from build123d import *

# Parameters (mm, degrees)
EXTRUDE1_DEPTH               = 10
EXTRUDE2_DEPTH               = 15
FILLET1_R                    = 8
SKETCH3_R                    = 2.5
CUT_EXTRUDE1_DEPTH           = 53.683044042
FILLET4_R                    = 8
FILLET7_R                    = 4
SKETCH4_W                    = 5
SKETCH4_H                    = 25.2
EXTRUDE3_DEPTH               = 117.395755978
F_4_0_4_DIAMETER_HOLE1_D     = 4
F_4_0_4_DIAMETER_HOLE1_DEPTH = 15
SKETCH6_W                    = 50
SKETCH6_H                    = 10
EXTRUDE4_DEPTH               = 22
SKETCH7_W                    = 35.991558426
SKETCH7_H                    = 19.258240123
EXTRUDE5_DEPTH               = 65
SKETCH8_R                    = 7
EXTRUDE6_DEPTH               = 65
SKETCH9_R                    = 11.25
EXTRUDE7_DEPTH               = 8
FILLET8_R                    = 10
SKETCH11_W                   = 10
SKETCH11_H                   = 24.2
EXTRUDE9_DEPTH               = 28
F_4_0_4_DIAMETER_HOLE2_D     = 4
F_4_0_4_DIAMETER_HOLE2_DEPTH = 15
SKETCH13_W                   = 8
SKETCH13_H                   = 22
CUT_EXTRUDE2_DEPTH           = 16
F_4_0_4_DIAMETER_HOLE3_D     = 3.9
F_4_0_4_DIAMETER_HOLE3_DEPTH = 15
EXTRUDE10_DEPTH              = 10
FILLET9_R                    = 5
FILLET10_R                   = 3


with BuildPart() as part:
    # Sketch1 → Extrude1 (new body)
    with BuildSketch(Plane.XY):
        Polygon((-68.067337579, -53.151608792), (46.932662421, -53.151608792), (46.932662421, -28.951608792), (56.08269406, -28.951608792), (56.08269406, -20.951608792), (46.932662421, -20.951608792), (46.932662421, 91.048391208), (36.605660332, 91.048391208), (25.932662421, 91.048391208), (25.932662421, 86.048391208), (36.932662421, 86.048391208), (36.932662421, 80.948391208), (25.932662421, 80.948391208), (25.932662421, 50.948391208), (36.932662421, 50.948391208), (36.932662421, 45.848391208), (25.932662421, 45.848391208), (25.932662421, 40.848391208), (36.932662421, 40.848391208), (36.932662421, 25.69350339), (36.932662421, 22.150468938), (36.932662421, 14.848391208), (-58.067337579, 14.848391208), (-58.067337579, -20.951608792), (-68.067337579, -20.951608792), align=None)
    extrude(amount=EXTRUDE1_DEPTH)

    # Sketch2 → Extrude2 (add)
    with BuildSketch(Plane.XY.offset(10)):
        Polygon((25.932662421, 91.048391208), (46.932662421, 91.048391208), (46.932662421, 41.227475545), (36.932662421, 41.227475545), (36.932662421, 40.848391208), (25.932662421, 40.848391208), (25.932662421, 45.848391208), (36.932662421, 45.848391208), (36.932662421, 50.948391208), (25.932662421, 50.948391208), (25.932662421, 80.948391208), (36.932662421, 80.948391208), (36.932662421, 86.048391208), (25.932662421, 86.048391208), align=None)
    extrude(amount=EXTRUDE2_DEPTH)

    # Fillet1
    fillet1_edges = [part.edges().sort_by_distance(p)[0] for p in [
        (25.932662421, 65.948391208, 0),
        (25.932662421, 65.948391208, 25),
    ]]
    fillet(fillet1_edges, radius=FILLET1_R)

    # Sketch3 → Cut-Extrude1 (cut)
    with BuildSketch(Plane(origin=(0, 91.048391208, 0), x_dir=(-1, 0, 0), z_dir=(0, 1, 0))):
        with Locations(Location((-30.932662421, 5.5, 0), (0, 0, 90))):
            Circle(SKETCH3_R)
        with Locations(Location((-30.932662421, 19.5, 0), (0, 0, 90))):
            Circle(SKETCH3_R)
    extrude(amount=-CUT_EXTRUDE1_DEPTH, mode=Mode.SUBTRACT)

    # Fillet4
    fillet4_edges = [part.edges().sort_by_distance(p)[0] for p in [
        (46.932662421, 91.048391208, 12.5),
    ]]
    fillet(fillet4_edges, radius=FILLET4_R)

    # Fillet7
    # the kernel refuses this fillet: 4 mm, written as the material it takes off along each edge
    with BuildSketch(Plane(origin=(46.932662421, 83.048391208, 25), x_dir=(-1, 0, 0), z_dir=(0, -1, 0))) as fillet7_piece_1:
        with BuildLine():
            CenterArc((FILLET7_R, FILLET7_R), FILLET7_R, 180, 90)
            Line((0, FILLET7_R), (0, 0))
            Line((0, 0), (FILLET7_R, 0))
        make_face()
    extrude(amount=51.820915662, mode=Mode.SUBTRACT)
    with BuildSketch(Plane(origin=(15.932662421, 91.048391208, 25), x_dir=(0, -1, 0), z_dir=(1, 0, 0))) as fillet7_piece_2:
        with BuildLine():
            CenterArc((FILLET7_R, FILLET7_R), FILLET7_R, 180, 90)
            Line((0, FILLET7_R), (0, 0))
            Line((0, 0), (FILLET7_R, 0))
        make_face()
    extrude(amount=23, mode=Mode.SUBTRACT)
    with BuildSketch(Plane(origin=(38.932662421, 83.048391208, 25), x_dir=(0, 1, 0), z_dir=(-1, 0, 0))) as fillet7_piece_3:
        with BuildLine():
            CenterArc((8 - FILLET7_R, FILLET7_R), FILLET7_R, 270, 90)
            Line((8, FILLET7_R), (8, 0))
            Line((8, 0), (8 - FILLET7_R, 0))
        make_face()
    revolve(axis=Axis((38.932662421, 83.048391208, 25), (0, 0, -1)), revolution_arc=90, mode=Mode.SUBTRACT)

    # Sketch4 → Extrude3 (cut, through all)
    with BuildSketch(Plane(origin=(0, 0, 0), x_dir=(-1, 0, 0), z_dir=(0, 0, -1))):
        with Locations((-44.432662421, 68.348391208)):
            Rectangle(SKETCH4_W, SKETCH4_H)
    extrude(amount=-EXTRUDE3_DEPTH, mode=Mode.SUBTRACT)

    # Ø4.0 (4) Diameter Hole1
    with Locations(Plane(origin=(41.932662421, 75.948391208, 12), x_dir=(0, 1, 0), z_dir=(1, 0, 0))):
        with Locations((0, 0), (-16, 0)):
            Hole(F_4_0_4_DIAMETER_HOLE1_D / 2, depth=F_4_0_4_DIAMETER_HOLE1_DEPTH)

    # Sketch6 → Extrude4 (add)
    with BuildSketch(Plane.XY.offset(10)):
        with Locations((-18.067337579, 9.848391208)):
            Rectangle(SKETCH6_W, SKETCH6_H)
    extrude(amount=EXTRUDE4_DEPTH)

    # Sketch7 → Extrude5 (cut)
    with BuildSketch(Plane.XY.offset(10)):
        with Locations((-17.995779213, -4.780728854)):
            Rectangle(SKETCH7_W, SKETCH7_H)
    extrude(amount=-EXTRUDE5_DEPTH, mode=Mode.SUBTRACT)

    # Sketch8 → Extrude6 (cut)
    with BuildSketch(Plane.XZ.offset(-4.848391208)):
        with Locations((-18.567337579, 16.771243445)):
            Circle(SKETCH8_R)
    extrude(amount=-EXTRUDE6_DEPTH, mode=Mode.SUBTRACT)

    # Sketch9 → Extrude7 (cut)
    with BuildSketch(Plane.XZ.offset(-4.848391208)):
        with Locations((-18.567337579, 16.771243445)):
            Circle(SKETCH9_R)
    extrude(amount=-EXTRUDE7_DEPTH, mode=Mode.SUBTRACT)

    # Fillet8
    fillet8_edges = [part.edges().sort_by_distance(p)[0] for p in [
        (6.932662421, 9.848391208, 32),
        (-43.067337579, 9.848391208, 32),
    ]]
    fillet(fillet8_edges, radius=FILLET8_R)

    # Sketch11 → Extrude9 (cut)
    with BuildSketch(Plane.XY.offset(10)):
        with Locations((-63.067337579, -41.051608792)):
            Rectangle(SKETCH11_W, SKETCH11_H)
    extrude(amount=-EXTRUDE9_DEPTH, mode=Mode.SUBTRACT)

    # Ø4.0 (4) Diameter Hole2
    with Locations(Plane(origin=(-63.067337579, -20.951608792, 5), x_dir=(1, 0, 0), z_dir=(0, 1, 0))):
        with Locations((0, 0), (114.57501582, 0)):
            Hole(F_4_0_4_DIAMETER_HOLE2_D / 2, depth=F_4_0_4_DIAMETER_HOLE2_DEPTH)

    # Sketch13 → Cut-Extrude2 (cut)
    with BuildSketch(Plane.XY.offset(10)):
        with Locations((-54.067337579, -0.049611207)):
            Rectangle(SKETCH13_W, SKETCH13_H)
    extrude(amount=-CUT_EXTRUDE2_DEPTH, mode=Mode.SUBTRACT)

    # Ø4.0 (4) Diameter Hole3
    with Locations(Plane(origin=(-50.067337579, 5.950388793, 5), x_dir=(0, 0, -1), z_dir=(-1, 0, 0))):
        with Locations((0, 0), (0, 12)):
            Hole(F_4_0_4_DIAMETER_HOLE3_D / 2, depth=F_4_0_4_DIAMETER_HOLE3_DEPTH)

    # Sketch10 → Extrude10 (cut)
    with BuildSketch(Plane.XY.offset(10)):
        Polygon((36.932662421, 4.848391208), (16.848954564, 4.848391208), (16.848954564, -4.813402299), (10.897809309, -4.813402299), (10.897809309, -24.409848915), (5.891741908, -24.409848915), (5.891741908, -43.151608792), (10.897809309, -43.151608792), (16.848954564, -43.151608792), (36.932662421, -43.151608792), align=None)
        Polygon((-43.449854697, -27.668574095), (-48.552654799, -27.668574095), (-48.552654799, -43.151608792), (-45.604016638, -43.151608792), (-3.328472946, -43.151608792), (-3.328472946, -24.409848915), (-43.449854697, -24.409848915), align=None)
    extrude(amount=-EXTRUDE10_DEPTH, mode=Mode.SUBTRACT)

    # Fillet9
    fillet9_edges = [part.edges().sort_by_distance(p)[0] for p in [
        (36.932662421, 4.848391208, 5),
        (36.932662421, -43.151608792, 5),
        (5.891741908, -43.151608792, 5),
        (5.891741908, -24.409848915, 5),
        (10.897809309, -4.813402299, 5),
        (16.848954564, 4.848391208, 5),
        (-3.328472946, -43.151608792, 5),
        (-48.552654799, -43.151608792, 5),
        (-48.552654799, -27.668574095, 5),
        (-3.328472946, -24.409848915, 5),
    ]]
    fillet(fillet9_edges, radius=FILLET9_R)

    # Fillet10
    fillet10_edges = [part.edges().sort_by_distance(p)[0] for p in [
        (-43.449854697, -26.039211505, 0),
        (16.848954564, -4.813402299, 5),
        (10.897809309, -24.409848915, 5),
    ]]
    fillet(fillet10_edges, radius=FILLET10_R)


solid = part.part
Build history of the part. All positions in model axes, mm. A direction names the side the tool comes from. Round coordinates to 2 decimals unless told otherwise and drop trailing zeros. Order: outer loops, then holes, each group sorted by start corner. A loop starts at its lowest first (then second) coordinate and runs counter-clockwise, first axis right, second up. Notation, with made-up numbers: M 48.25,45 L 68.25,45 A31 cw 68.25,79 Z; hole C 16,-15 d8. An arc over 180 degrees is marked long. Use CSV: the item, a comma, the result in double quotes. Start each with the question number.
(1) Tool access for faces 4 (the face through (29.98, 88.58, 7.81)), 5 (the face through (28.21, 65.74, 2.41)), 6 (the face through (-35.067, 6, 5)): list every direction of +Z, -Z, +X, -X, +Y, -Y with a clear straight run to the whole face (end or side of a thin tool).
(2) Cut at B-B on y = 33.5. List the corners of the cut face in (x, z), then the cut area to 3 significant figures.
(3) Mould opens along X. For faces 1 (the face through (-4.754, -25.913, 4.93)), 2 (the face through (-40.22, 9.92, 28.99)), 3 (the face through (54, -20.952, 5)) say: +X half, -X half, draft (parallel to the pull), parting line (faces both ways), or undercut.
(4) Flat gauge pins, fed straight in: P1, Ø7, axis at y = -33.5, z = 6, coming from the -X side; P2, Ø8, axis at x = -64.5, z = 3, coming from the -Y side; P3, Ø8, axis at x = -48.5, y = -22.5, coming from the +Z side; P4, Ø6.5, axis at x = 30.93, z = 5.5, coming from the +Y side. Where does each tip first touch, or does it go through?
(5) Cut at A-A on x = -39. List the corners of the cut face in (y, z), then the cut area to 3 significant figures.
(6) Drill centre lines: probe 1 along Y at (x, z) = (28, 20.5); probe 2 along X at (y, z) = (-42, 2); probe 3 along Y at (x, z) = (33, 7). Where is each one in solid material? Low to high.
(7) Cut at C-C on z = 12. State how many separate pieces and enclosed holes the cut face has, then the cut area to 3 significant figures.
Findings:
1,face 4,"+Y"
1,face 5,"-Z, -X"
1,face 6,"-X"
2,outline,"M 36.93,0 L 46.93,0 L 46.93,10 L 36.93,10 Z"
2,area,"100 mm^2"
3,face 1,"undercut"
3,face 2,"-X half"
3,face 3,"draft"
4,P1,"stops at x = -58.07"
4,P2,"stops at y = -28.95"
4,P3,"stops at z = 10"
4,P4,"stops at y = 91.05"
5,outline,"M -53.15,0 L -43.15,0 L -43.15,10 L -53.15,10 Z; M -24.41,0 L 14.85,0 L 14.85,30.05 L 4.85,30.05 L 4.85,10 L -24.41,10 Z; hole C -6.05,5 d3.9; hole C 5.95,5 d3.9"
5,area,"669 mm^2"
6,probe 1,"y = 40.85 to 45.85, 50.95 to 80.95, 86.05 to 91.05"
6,probe 2,"x = -58.07 to -46.74, -5.14 to 7.7, 35.12 to 46.93"
6,probe 3,"y = -53.15 to -43.04, 4.73 to 14.85, 40.85 to 45.85, 50.95 to 80.95, 86.05 to 91.05"
7,separate pieces,"3"
7,enclosed holes,"0"
7,area,"995 mm^2"
